Check sheet for the modelled part. Datum: model origin and axes. Units: mm. Face numbers are marked on the shaded views. A direction names the side the tool comes from. Coordinates: 2 decimals unless noted, no trailing zeros. Order: outer loops, then holes, each group sorted by start corner. A loop starts at its lowest first (then second) coordinate and runs counter-clockwise, first axis right, second up.
1. Set-up check for the marked faces 1 and 2: record each of +Z, -Z, +X, -X, +Y, -Y from which the full face is reachable in a straight line by a thin tool's end or side.
2. Cross-section at A-A (y = -63.5). Count the separate pieces of the cut face and the enclosed holes in it, then the cut area to 3 significant figures.
3. Gauge pin test, flat ends, axial feed: pin 1 Ø3.5 at (x, z) = (-51, 3.5) entering from +Y; pin 2 Ø4 at (x, y) = (-21.59, -25.4) entering from +Z. Record the tip position at first contact, or that the pin passes through.
4. Cross-section at D-D (y = -82.55). Enter the section's corners in (x, z), then the cut area to 3 significant figures.
5. Cross-section at B-B (x = -42). Enter the section's corners in (y, z).
6. Thickness scan on line 1 (Y direction, x = -21.59, z = 6); line 2 (X direction, y = -6.35, z = 9); line 3 (X direction, y = -43.5, z = 8.25). Record the ranges inside material, lowest first.
7. Draft check along Z on the marked faces 3, 4 and 5. Enter one of: released by +Z, released by -Z, zero draft, split by the parting line, or undercut.
```python
from build123d import *

# Parameters (mm, degrees)
F1_DEPTH = 88.9
F2_W     = 4.9823306459
F2_H     = 18.9774408937
F3_DEPTH = 127
F4_R     = 1.5875
F5_DEPTH = 127
F6_R     = 1.4161925478
F6_R_2   = 1.5875
F7_DEPTH = 76.2


with BuildPart() as f1:
    # F0 (on Front) → F1 (new body)
    with BuildSketch(Plane.XZ):
        with BuildLine():
            Line((-22.8439420462, 0), (0, 0))
            Line((0, 0), (0, 17.765391618))
            Line((0, 17.765391618), (-4.1987905279, 17.765391618))
            Line((-4.1987905279, 17.765391618), (-4.1987905279, 16.4750870317))
            Line((-4.1987905279, 16.4750870317), (-4.1987905279, 15.044271946))
            Line((-4.1987905279, 15.044271946), (-4.1987905279, 9.3032421722))
            ThreePointArc((-4.1987905279, 9.3032421722), (-9.6494707531, 3.097937748), (-15.1226427406, 9.2834131792))
            Line((-15.1226427406, 9.2834131792), (-15.1226427406, 15.044271946))
            Line((-15.1226427406, 15.044271946), (-15.1226427406, 16.4750870317))
            Line((-15.1226427406, 16.4750870317), (-15.1226427406, 17.765391618))
            Line((-15.1226427406, 17.765391618), (-16.0616673529, 17.765391618))
            Line((-16.0616673529, 17.765391618), (-16.0616673529, 11.8045024574))
            Line((-16.0616673529, 11.8045024574), (-18.7766868621, 11.8045024574))
            Line((-18.7766868621, 11.8045024574), (-63.7612715364, 11.8045024574))
            Line((-63.7612715364, 11.8045024574), (-66.2720091641, 11.8045024574))
            Line((-66.2720091641, 11.8045024574), (-66.2720091641, 17.765391618))
            Line((-66.2720091641, 17.765391618), (-67.2196410596, 17.765391618))
            Line((-67.2196410596, 17.765391618), (-67.2196410596, 16.4750870317))
            Line((-67.2196410596, 16.4750870317), (-67.2196410596, 15.044271946))
            Line((-67.2196410596, 15.044271946), (-67.2196410596, 9.2371329665))
            ThreePointArc((-67.2196410596, 9.2371329665), (-72.6834610105, 3.0635382866), (-78.1472809613, 9.2371329665))
            Line((-78.1472809613, 9.2371329665), (-78.1472809613, 15.044271946))
            Line((-78.1472809613, 15.044271946), (-78.1472809613, 16.4750870317))
            Line((-78.1472809613, 16.4750870317), (-78.1472809613, 17.765391618))
            Line((-78.1472809613, 17.765391618), (-82.3283270001, 17.765391618))
            Line((-82.3283270001, 17.765391618), (-82.3283270001, 0))
            Line((-82.3283270001, 0), (-22.8439420462, 0))
        make_face()
        with BuildLine():
            Line((-4.1987905279, 16.4750870317), (-4.1987905279, 17.765391618))
            ThreePointArc((-4.1987905279, 17.765391618), (-5.5930091509, 16.810932091), (-7.2489217855, 16.4750870317))
            Line((-7.2489217855, 16.4750870317), (-4.1987905279, 16.4750870317))
        make_face()
        Polygon((-4.1987905279, 15.044271946), (-4.1987905279, 16.4750870317), (-7.2489217855, 16.4750870317), align=None)
        with BuildLine():
            ThreePointArc((-75.1015543938, 16.4750870317), (-76.755438931, 16.8109674547), (-78.1472809613, 17.765391618))
            Line((-78.1472809613, 17.765391618), (-78.1472809613, 16.4750870317))
            Line((-78.1472809613, 16.4750870317), (-75.1015543938, 16.4750870317))
        make_face()
        Polygon((-75.1015543938, 16.4750870317), (-78.1472809613, 16.4750870317), (-78.1472809613, 15.044271946), align=None)
        Polygon((-15.1226427406, 16.4750870317), (-15.1226427406, 15.044271946), (-12.0709454641, 16.4750870317), align=None)
        with BuildLine():
            Line((-15.1226427406, 17.765391618), (-15.1226427406, 16.4750870317))
            Line((-15.1226427406, 16.4750870317), (-12.0709454641, 16.4750870317))
            ThreePointArc((-12.0709454641, 16.4750870317), (-13.7275792644, 16.8109195511), (-15.1226427406, 17.765391618))
        make_face()
        Polygon((-70.2685788274, 16.4750870317), (-67.2196410596, 15.044271946), (-67.2196410596, 16.4750870317), align=None)
        with BuildLine():
            Line((-16.0616673529, 11.8045024574), (-16.0616673529, 17.765391618))
            ThreePointArc((-16.0616673529, 17.765391618), (-16.7723874031, 14.4903522854), (-18.7766868621, 11.8045024574))
            Line((-18.7766868621, 11.8045024574), (-16.0616673529, 11.8045024574))
        make_face()
        with BuildLine():
            Line((-70.2685788274, 16.4750870317), (-67.2196410596, 16.4750870317))
            Line((-67.2196410596, 16.4750870317), (-67.2196410596, 17.765391618))
            ThreePointArc((-67.2196410596, 17.765391618), (-68.6132157677, 16.8109416595), (-70.2685788274, 16.4750870317))
        make_face()
        with BuildLine():
            Line((-66.2720091641, 11.8045024574), (-63.7612715364, 11.8045024574))
            ThreePointArc((-63.7612715364, 11.8045024574), (-65.6187109531, 14.5313537773), (-66.2720091641, 17.765391618))
            Line((-66.2720091641, 17.765391618), (-66.2720091641, 11.8045024574))
        make_face()
    extrude(amount=F1_DEPTH)

    # F2 (on Top) → F3 (cut)
    with BuildSketch(Plane.XY):
        Polygon((-30.48, -12.7), (-60.96, -12.7), (-60.96, -76.2), (-30.48, -76.2), (-30.48, -52.5795705616), (-30.48, -33.602129668), align=None)
        with Locations((-27.988834677, -43.0908501148)):
            Rectangle(F2_W, F2_H)
    extrude(amount=F3_DEPTH, mode=Mode.SUBTRACT)

    # F4 (on Top) → F5 (cut)
    with BuildSketch(Plane.XY):
        with Locations((-21.59, -25.4)):
            Circle(F4_R)
        with Locations((-21.59, -63.5)):
            Circle(F4_R)
    extrude(amount=F5_DEPTH, mode=Mode.SUBTRACT)

    # F6 (on Top) → F7 (cut)
    with BuildSketch(Plane.XY):
        with Locations((-50.8, -6.35)):
            Circle(F6_R)
        with Locations((-50.7999993861, -82.55)):
            Circle(F6_R_2)
    extrude(amount=F7_DEPTH, mode=Mode.SUBTRACT)


solid = f1.part
```
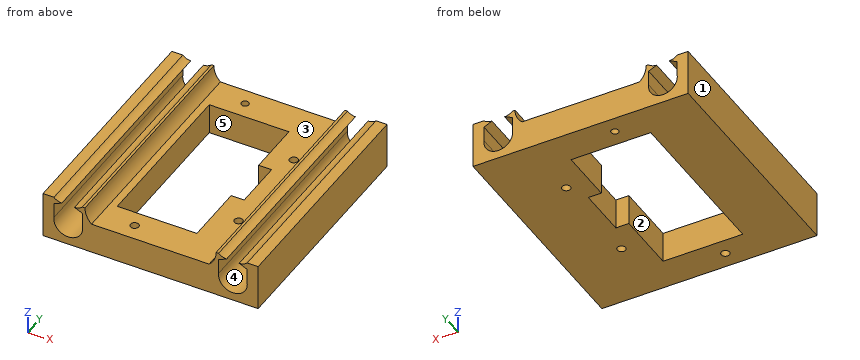
Data:
1. face 1: +Z, -Z, -X, +Y, -Y
1. face 2: +Z, -Z
2. separate pieces: 3
2. enclosed holes: 0
2. area: 493 mm2
3. pin 1: stops at y = 0
3. pin 2: stops at z = 11.8
4. outline: (-82.33, 0) - (-52.39, 0) - (-52.39, 11.8) - (-63.76, 11.8) arc R8.33 cw to (-66.27, 17.77) - (-67.22, 17.77) arc R4.25 cw to (-70.27, 16.48) - (-67.22, 15.04) - (-67.22, 9.24) arc R5.5 cw (long way) to (-78.15, 9.24) - (-78.15, 15.04) - (-75.1, 16.48) arc R4.24 cw to (-78.15, 17.77) - (-82.33, 17.77) - close; (-49.21, 0) - (0, 0) - (0, 17.77) - (-4.2, 17.77) arc R4.25 cw to (-7.25, 16.48) - (-4.2, 15.04) - (-4.2, 9.3) arc R5.51 cw (long way) to (-15.12, 9.28) - (-15.12, 15.04) - (-12.07, 16.48) arc R4.25 cw to (-15.12, 17.77) - (-16.06, 17.77) arc R7.9 cw to (-18.78, 11.8) - (-49.21, 11.8) - close
4. area: 853 mm2
5. outline: (-88.9, 0) - (-76.2, 0) - (-76.2, 11.8) - (-88.9, 11.8) - close; (-12.7, 0) - (0, 0) - (0, 11.8) - (-12.7, 11.8) - close
6. line 1: y = -88.9 to -65.09, -61.91 to -26.99, -23.81 to 0
6. line 2: x = -82.33 to -78.17, -67.2 to -52.22, -49.38 to -15.15, -4.17 to 0
6. line 3: x = -82.33 to -78.18, -67.19 to -60.96, -25.5 to -15.15, -4.17 to 0
7. face 3: released by +Z
7. face 4: undercut
7. face 5: zero draft
